The listing builds one solid part. Answer for the finished solid, in the listing's coordinates (mm). Face numbers are marked on the shaded views. A direction names the side the tool comes from. Coordinates: 2 decimals unless noted, no trailing zeros. Write each loop counter-clockwise with the first axis right and the second up, starting at its lowest first coordinate (ties: lowest second). Pieces come first, ordered by that corner, then holes.
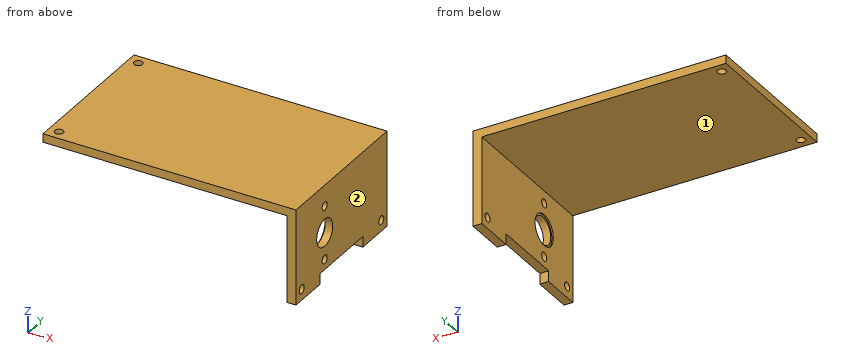
from build123d import *

# Parameters (mm, degrees)
BOSS_EXTRUDE1_DEPTH = 54.9
SKETCH2_R           = 1.51
CUT_EXTRUDE1_DEPTH  = 3.15
SKETCH3_R           = 1.51
CUT_EXTRUDE2_DEPTH  = 3
SKETCH4_R           = 4.826
SKETCH4_R_2         = 1.515
CUT_EXTRUDE3_DEPTH  = 3.15
SKETCH6_R           = 5.5
CUT_EXTRUDE5_DEPTH  = 0.5
SKETCH8_W           = 3.798879325
SKETCH8_H           = 25.75548204
CUT_EXTRUDE7_DEPTH  = 3.15


with BuildPart() as part:
    # Sketch1 → Boss-Extrude1 (new body)
    with BuildSketch(Plane(origin=(0, 0, 0), x_dir=(1, 0, 0), z_dir=(0, 1, 0))):
        Polygon((0, 0), (86.85, 0), (86.85, 30.9), (90, 30.9), (90, -3), (0, -3), align=None)
    extrude(amount=BOSS_EXTRUDE1_DEPTH)

    # Sketch2 → Cut-Extrude1 (cut)
    with BuildSketch(Plane(origin=(90, 0, 0), x_dir=(0, 0, -1), z_dir=(1, 0, 0))):
        with Locations((27, 51.45)):
            Circle(SKETCH2_R)
        with Locations((27, 3.45)):
            Circle(SKETCH2_R)
    extrude(amount=-CUT_EXTRUDE1_DEPTH, mode=Mode.SUBTRACT)

    # Sketch3 → Cut-Extrude2 (cut)
    with BuildSketch(Plane.XY.offset(3)):
        with Locations((3.625, 51.325)):
            Circle(SKETCH3_R)
        with Locations((3.625, 3.575)):
            Circle(SKETCH3_R)
    extrude(amount=-CUT_EXTRUDE2_DEPTH, mode=Mode.SUBTRACT)

    # Sketch4 → Cut-Extrude3 (cut)
    with BuildSketch(Plane(origin=(90, 0, 0), x_dir=(0, 0, -1), z_dir=(1, 0, 0))):
        with Locations((13.95544469, 17.3)):
            Circle(SKETCH4_R)
        with Locations((23.45544469, 17.3)):
            Circle(SKETCH4_R_2)
        with Locations((4.45544469, 17.3)):
            Circle(SKETCH4_R_2)
    extrude(amount=-CUT_EXTRUDE3_DEPTH, mode=Mode.SUBTRACT)

    # Sketch6 → Cut-Extrude5 (cut)
    with BuildSketch(Plane.ZY.offset(-86.85)):
        with Locations((-13.95544469, 17.3)):
            Circle(SKETCH6_R)
    extrude(amount=-CUT_EXTRUDE5_DEPTH, mode=Mode.SUBTRACT)

    # Sketch8 → Cut-Extrude7 (cut)
    with BuildSketch(Plane(origin=(90, 0, 0), x_dir=(0, 0, -1), z_dir=(1, 0, 0))):
        with Locations((29.000560338, 27.45)):
            Rectangle(SKETCH8_W, SKETCH8_H)
    extrude(amount=-CUT_EXTRUDE7_DEPTH, mode=Mode.SUBTRACT)


solid = part.part
1. Section C-C on y = 44.5 is taken. Give the vertices of the cut face in (x, z).
Results found:
outline: (0, 0) - (86.85, 0) - (86.85, -30.9) - (90, -30.9) - (90, 3) - (0, 3) - close
2. Find the intervals of material crossed by L1, parallel to Z at x = 89, y = 17; L2, parallel to X at y = 45.5, z = -2.5; L3, parallel to Z at x = 15.5, y = 41, in increasing order.
Results found:
L1: z = -27.1 to -24.94, -21.97 to -18.77, -9.14 to -5.94, -2.97 to 3
L2: x = 86.85 to 90
L3: z = 0 to 3
3. Flat-ended cylindrical pins translate along their axes: P1, Ø16.5, axis at x = 48.5, y = 34, coming from the -Z side; P2, Ø2.5, axis at x = 3.625, y = 51.325, coming from the +Z side; P3, Ø12, axis at y = 15, z = -12.5, coming from the -X side; P4, Ø1.6, axis at x = 89, y = 28, coming from the -Z side. Find the tip coordinate at first contact, or state that the pin passes through.
Results found:
P1: stops at z = 0
P2: passes through
P3: stops at x = 86.85
P4: stops at z = -27.1
4. Section B-B on z = -15.5 is taken. Give the vertices of the cut face in (x, y), then the cut area to 3 significant figures.
Results found:
outline: (86.85, 0) - (90, 0) - (90, 12.73) - (87.35, 12.73) - (87.35, 12.02) - (86.85, 12.02) - close; (86.85, 22.58) - (87.35, 22.58) - (87.35, 21.87) - (90, 21.87) - (90, 54.9) - (86.85, 54.9) - close
area: 143 mm2
5. A tool of negligible diameter and unlimited length cuts with its end or side. For the marked faces 1 and 2, from which of +Z, -Z, +X, -X, +Y, -Y can it reach the whole face along a straight path? Write none if from no direction.
Results found:
face 1: -Z, -X, +Y, -Y
face 2: +Z, -Z, +X, +Y, -Y
6. Section A-A on y = 17.3 is taken. Give the vertices of the cut face in (x, z).
Results found:
outline: (0, 0) - (86.85, 0) - (86.85, -2.94) - (90, -2.94) - (90, 3) - (0, 3) - close; (86.85, -27.1) - (90, -27.1) - (90, -24.97) - (86.85, -24.97) - close; (86.85, -21.94) - (90, -21.94) - (90, -18.78) - (87.35, -18.78) - (87.35, -19.46) - (86.85, -19.46) - close; (86.85, -8.46) - (87.35, -8.46) - (87.35, -9.13) - (90, -9.13) - (90, -5.97) - (86.85, -5.97) - close
7. Section D-D on z = -7.5 is taken. Give the vertices of the cut face in (x, y), then the cut area to 3 significant figures.
Results found:
outline: (86.85, 0) - (90, 0) - (90, 54.9) - (86.85, 54.9) - close
area: 173 mm2
